from build123d import *

# Parameters (mm, degrees)
SKETCH1_W           = 5
SKETCH1_H           = 5
BOSS_EXTRUDE1_DEPTH = 1
SKETCH2_W           = 0.7
SKETCH2_H           = 0.7
BOSS_EXTRUDE2_DEPTH = 0.5
SKETCH7_W           = 0.7
SKETCH7_H           = 0.5
BOSS_EXTRUDE3_DEPTH = 3
SKETCH8_W           = 0.7
SKETCH8_H           = 0.7
BOSS_EXTRUDE4_DEPTH = 0.5
SKETCH9_W           = 0.7
SKETCH9_H           = 0.5
BOSS_EXTRUDE5_DEPTH = 3


with BuildPart() as part:
    # Sketch1 → Boss-Extrude1 (new body)
    with BuildSketch(Plane(origin=(0, 0, 0), x_dir=(1, 0, 0), z_dir=(0, 1, 0))):
        Rectangle(SKETCH1_W, SKETCH1_H)
    extrude(amount=BOSS_EXTRUDE1_DEPTH)

    # Sketch2 → Boss-Extrude2 (add)
    with BuildSketch(Plane.XY.offset(2.5)):
        with Locations((-1.85, 0.5)):
            Rectangle(SKETCH2_W, SKETCH2_H)
        with Locations((1.85, 0.5)):
            Rectangle(SKETCH2_W, SKETCH2_H)
    extrude(amount=BOSS_EXTRUDE2_DEPTH)

    # Sketch7 → Boss-Extrude3 (add)
    with BuildSketch(Plane(origin=(0, 0.85, 0), x_dir=(1, 0, 0), z_dir=(0, 1, 0))):
        with Locations((-1.85, -3)):
            Rectangle(SKETCH7_W, SKETCH7_H)
        with Locations((1.85, -3)):
            Rectangle(SKETCH7_W, SKETCH7_H)
    extrude(amount=-BOSS_EXTRUDE3_DEPTH)

    # Sketch8 → Boss-Extrude4 (add)
    with BuildSketch(Plane(origin=(0, 0, -2.5), x_dir=(-1, 0, 0), z_dir=(0, 0, -1))):
        with Locations((-1.85, 0.5)):
            Rectangle(SKETCH8_W, SKETCH8_H)
        with Locations((1.85, 0.5)):
            Rectangle(SKETCH8_W, SKETCH8_H)
    extrude(amount=BOSS_EXTRUDE4_DEPTH)

    # Sketch9 → Boss-Extrude5 (add)
    with BuildSketch(Plane(origin=(0, 0.85, 0), x_dir=(1, 0, 0), z_dir=(0, 1, 0))):
        with Locations((-1.85, 3)):
            Rectangle(SKETCH9_W, SKETCH9_H)
        with Locations((1.85, 3)):
            Rectangle(SKETCH9_W, SKETCH9_H)
    extrude(amount=-BOSS_EXTRUDE5_DEPTH)


solid = part.part
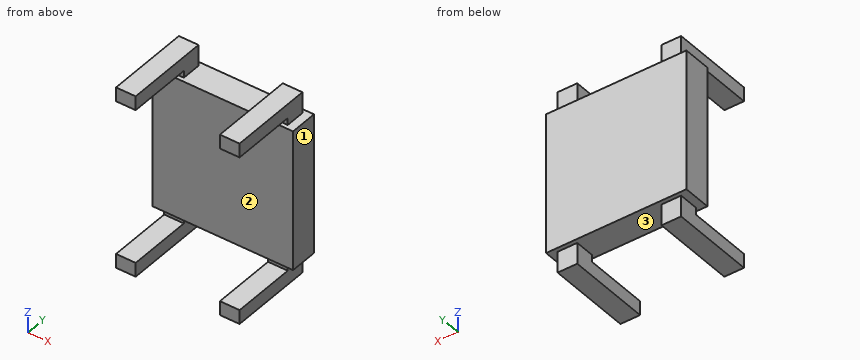
Build history of the part. All positions in model axes, mm. Face numbers are marked on the shaded views. Round coordinates to 2 decimals unless told otherwise and drop trailing zeros. Loops run counter-clockwise (first coordinate to the right, second up) from the corner with the lowest first, then second, coordinate; pieces in that order, holes last. Notation, with made-up numbers: (28.5, 40.5) -> (66.5, 40.5) arc R21 cw to (66.5, 74.5) -> close; hole circle Ø5 at (19, 24). An arc over 180 degrees is marked (long way). Answer in a Markdown table with one row per item.
Item 1: Saw through at C-C (z = -1.5). Write the cut outline in (x, y), and give its area (3 significant figures).
Answers below:
| item | result |
|---|---|
| outline | (-2.5, 0) -> (2.5, 0) -> (2.5, 1) -> (-2.5, 1) -> close |
| area | 5.00 mm² |
Item 2: Pin check, flat tips, straight feed: pin 1 (0.5 mm diameter, centred on x = -0.5, y = 0.5, fed in from -Z); pin 2 (0.8 mm diameter, centred on x = -2, z = 3, fed in from +Y); pin 3 (0.6 mm diameter, centred on y = -0.5, z = 3, fed in from -X); pin 4 (1.5 mm diameter, centred on x = 0.5, y = -1, fed in from -Z). Stop position of each tip, or through.
Answers below:
| item | result |
|---|---|
| pin 1 | stops at z = -2.5 |
| pin 2 | stops at y = 0.85 |
| pin 3 | stops at x = -2.2 |
| pin 4 | passes through |
Item 3: Mould opens along X. For the marked faces 1, 2 and 3 say: +X half, -X half, draft (parallel to the pull), parting line (faces both ways), or undercut.
Answers below:
| item | result |
|---|---|
| face 1 | +X half |
| face 2 | draft |
| face 3 | undercut |
Item 4: Saw through at B-B (x = -1.75). Write the cut outline in (y, z), and give its area (3 significant figures).
Answers below:
| item | result |
|---|---|
| outline | (-2.15, -3.25) -> (0.85, -3.25) -> (0.85, -2.5) -> (1, -2.5) -> (1, 2.5) -> (0.85, 2.5) -> (0.85, 3.25) -> (-2.15, 3.25) -> (-2.15, 2.75) -> (0.15, 2.75) -> (0.15, 2.5) -> (0, 2.5) -> (0, -2.5) -> (0.15, -2.5) -> (0.15, -2.75) -> (-2.15, -2.75) -> close |
| area | 8.35 mm² |
Item 5: Saw through at D-D (x = -0.35). Write the cut outline in (y, z), and give its area (3 significant figures).
Answers below:
| item | result |
|---|---|
| outline | (0, -2.5) -> (1, -2.5) -> (1, 2.5) -> (0, 2.5) -> close |
| area | 5.00 mm² |
Item 6: Drill centre lines: L1, parallel to X at y = -2, z = 3; L2, parallel to Y at x = 0.8, z = 1.75; L3, parallel to Z at x = 0, y = 0.4. Where is each one in solid material? Low to high. Write a range as [from, to].
Answers below:
| item | result |
|---|---|
| L1 | x = [-2.2, -1.5], [1.5, 2.2] |
| L2 | y = [0, 1] |
| L3 | z = [-2.5, 2.5] |
Item 7: Saw through at A-A (y = -0.1). Write the cut outline in (x, z).
Answers below:
| item | result |
|---|---|
| outline | (-2.2, -3.25) -> (-1.5, -3.25) -> (-1.5, -2.75) -> (-2.2, -2.75) -> close; (-2.2, 2.75) -> (-1.5, 2.75) -> (-1.5, 3.25) -> (-2.2, 3.25) -> close; (1.5, -3.25) -> (2.2, -3.25) -> (2.2, -2.75) -> (1.5, -2.75) -> close; (1.5, 2.75) -> (2.2, 2.75) -> (2.2, 3.25) -> (1.5, 3.25) -> close |
